Design review of the part built by this model. Coordinates are the model's own, in mm. A direction names the side the tool comes from. Give positions to 0.01 mm unless a question says otherwise; leave off trailing zeros. Write each loop counter-clockwise with the first axis right and the second up, starting at its lowest first coordinate (ties: lowest second). Pieces come first, ordered by that corner, then holes.
```python
from build123d import *

# Parameters (mm, degrees)
F1_DEPTH = 3
F2_R     = 5
F2_R_2   = 2.75
F3_DEPTH = 3
F4_R     = 2.25
F5_DEPTH = 3
F6_R     = 1


with BuildPart() as f1:
    # F0 (on Top) → F1 (new body)
    with BuildSketch(Plane.XY):
        with BuildLine():
            ThreePointArc((25, 48), (24.414214, 49.414214), (23, 50))
            Line((23, 50), (-23, 50))
            ThreePointArc((-23, 50), (-24.414214, 49.414214), (-25, 48))
            Line((-25, 48), (-25, -48))
            ThreePointArc((-25, -48), (-24.414214, -49.414214), (-23, -50))
            Line((-23, -50), (-21.25, -50))
            ThreePointArc((-21.25, -50), (-17.714466, -51.464466), (-16.25, -55))
            Line((-16.25, -55), (-16.25, -86))
            Line((-16.25, -86), (0, -86))
            Line((0, -86), (16.25, -86))
            Line((16.25, -86), (16.25, -55))
            ThreePointArc((16.25, -55), (17.714466, -51.464466), (21.25, -50))
            Line((21.25, -50), (23, -50))
            ThreePointArc((23, -50), (24.414214, -49.414214), (25, -48))
            Line((25, -48), (25, 48))
        make_face()
    extrude(amount=F1_DEPTH)

    # F2 (on face) → F3 (cut, through all)
    with BuildSketch(Plane.XY.offset(3)):
        with Locations((-10, -25)):
            Circle(F2_R)
        with Locations((-10, 0)):
            Circle(F2_R_2)
        with Locations((-10, 25)):
            Circle(F2_R_2)
        with Locations((10, 25)):
            Circle(F2_R_2)
        with Locations((10, 0)):
            Circle(F2_R_2)
        with Locations((10, -25)):
            Circle(F2_R)
    extrude(amount=-F3_DEPTH, mode=Mode.SUBTRACT)

    # F4 (on face) → F5 (cut, through all)
    with BuildSketch(Plane.XY.offset(3)):
        with Locations((-9, -60)):
            Circle(F4_R)
        with Locations((9, -60)):
            Circle(F4_R)
        with Locations((9, -78)):
            Circle(F4_R)
        with Locations((-9, -78)):
            Circle(F4_R)
    extrude(amount=-F5_DEPTH, mode=Mode.SUBTRACT)

    # F6
    f6_edges = [f1.edges().sort_by_distance(p)[0] for p in [
        (-16.25, -86, 1.5),
        (16.25, -86, 1.5),
    ]]
    fillet(f6_edges, radius=F6_R)


solid = f1.part
```
(1) Consider section C-C, the plane z = 0.5. Give the number of separate pieces and of enclosed holes in the cut face, then the cut area to 3 significant figures.
Resolved:
separate pieces: 1
enclosed holes: 10
area: 5,860 mm2
(2) Consider section D-D, the plane y = -60. Give the boundary of the cut face in (x, z), then the cut area to 3 significant figures.
Resolved:
outline: (-16.25, 0) - (-11.25, 0) - (-11.25, 3) - (-16.25, 3) - close; (-6.75, 0) - (6.75, 0) - (6.75, 3) - (-6.75, 3) - close; (11.25, 0) - (16.25, 0) - (16.25, 3) - (11.25, 3) - close
area: 70.5 mm2
(3) Clearance check with flat-ended pins moving along their axes: P1, Ø3.5, axis at x = 10, y = 0, coming from the -Z side; P2, Ø1.4, axis at x = -21.5, z = 1.5, coming from the -Y side; P3, Ø1.5, axis at y = -49.5, z = 2, coming from the -X side; P4, Ø0.9, axis at y = -66.5, z = 2, coming from the -X side. State where each tip first meets the part, or that it passes through.
Resolved:
P1: passes through
P2: stops at y = -50.02
P3: stops at x = -24.85
P4: stops at x = -16.25
(4) Consider section A-A, the plane y = -25. Give the boundary of the cut face in (x, z), then the cut area to 3 significant figures.
Resolved:
outline: (-25, 0) - (-15, 0) - (-15, 3) - (-25, 3) - close; (-5, 0) - (5, 0) - (5, 3) - (-5, 3) - close; (15, 0) - (25, 0) - (25, 3) - (15, 3) - close
area: 90.0 mm2
(5) To check wall thickness, follow L1, parallel to Y at x = -10.5, z = 0.8; L2, parallel to Y at x = 9, z = 2; L3, parallel to X at y = -75.5, z = 0.6. State the ranges of each line that lie inside material, in increasing order.
Resolved:
L1: y = -86 to -79.68, -76.32 to -61.68, -58.32 to -29.97, -20.03 to -2.7, 2.7 to 22.3, 27.7 to 50
L2: y = -86 to -80.25, -75.75 to -62.25, -57.75 to -29.9, -20.1 to -2.56, 2.56 to 22.44, 27.56 to 50
L3: x = -16.25 to 16.25
(6) Mouldability with a two-part tool opening along X and no side actions: class faces 1 (the face through (17.68, -51.5, 1.48)), 2 (the face through (-10.786, -61.369, 1.521)), 3 (the face through (0, -86, 1)) as pulls with the +X half, pulls with the -X half, needs draft (parallel to the pull), parting line crosses it, or undercut.
Resolved:
face 1: pulls with the +X half
face 2: undercut
face 3: needs draft
(7) Tool access review of faces 4 (the face through (16.25, -70, 1)), 5 (the face through (12.54, -1.05, 1.52)): name each direction out of +Z, -Z, +X, -X, +Y, -Y from which nothing blocks a thin tool from reaching the whole face with its end or side.
Resolved:
face 4: +Z, -Z, +X, -Y
face 5: +Z, -Z
(8) Consider section B-B, the plane x = -10. Give the boundary of the cut face in (y, z).
Resolved:
outline: (-86, 0) - (-80.02, 0) - (-80.02, 3) - (-86, 3) - close; (-75.98, 0) - (-62.02, 0) - (-62.02, 3) - (-75.98, 3) - close; (-57.98, 0) - (-30, 0) - (-30, 3) - (-57.98, 3) - close; (-20, 0) - (-2.75, 0) - (-2.75, 3) - (-20, 3) - close; (2.75, 0) - (22.25, 0) - (22.25, 3) - (2.75, 3) - close; (27.75, 0) - (50, 0) - (50, 3) - (27.75, 3) - close
